Can you work these out from the model? Positions are in its coordinate system, mm. Face numbers are marked on the shaded views. A direction names the side the tool comes from. Round coordinates to 2 decimals unless told otherwise and drop trailing zeros. Write each loop counter-clockwise with the first axis right and the second up, starting at its lowest first coordinate (ties: lowest second). Pieces come first, ordered by that corner, then holes. Notation, with made-up numbers: M 79.25,8 L 97.25,8 A17 cw 97.25,41 Z; hole C 57,61.25 d10. An arc over 180 degrees is marked long. Answer in a Markdown table with one row per item. Add a question column.
(1) I'm going to push flat-ended pins straight in: pin 1 (2 mm diameter, centred on y = 4, z = -3, fed in from +X); pin 2 (1.5 mm diameter, centred on x = 15.5, z = -2, fed in from +Y); pin 3 (1.5 mm diameter, centred on x = 15, z = -3.5, fed in from -Y); pin 4 (1.5 mm diameter, centred on y = 5.5, z = -4, fed in from -X). Where does each tip first touch, or does it pass through?
(2) Suppose I cut it at A-A, the plane y = 0. Write out the boundary of the cut face in (x, z), then the cut area to 3 significant figures.
(3) For the marked faces 1, 2, 3, 4 and 5, which set-ups out of +Z, -Z, +X, -X, +Y, -Y let a thin tool reach every point of the face, with its end or its side?
(4) If we mould it in two halves opening along Y, with no side actions, what happens to the marked faces 6, 7 and 8? For each: released by +Y, released by -Y, zero draft, split by the parting line, or undercut.
(5) Suppose I cut it at D-D, the plane x = 8.5. Write out the boundary of the cut face in (y, z), then the cut area to 3 significant figures.
(6) Suppose I cut it at B-B, the plane x = 14.5. Write out the boundary of the cut face in (y, z), then the cut area to 3 significant figures.
(7) Suppose I cut it at C-C, the plane z = -2.56. Write out the boundary of the cut face in (x, y).
(8) If I drill on probe 1 along Y at (x, z) = (16.5, -3.6); probe 2 along X at (y, z) = (-3.6, -2.56); probe 3 along Z at (x, y) = (8, 2), over which ranges is the centre line in solid material (lowest first)?
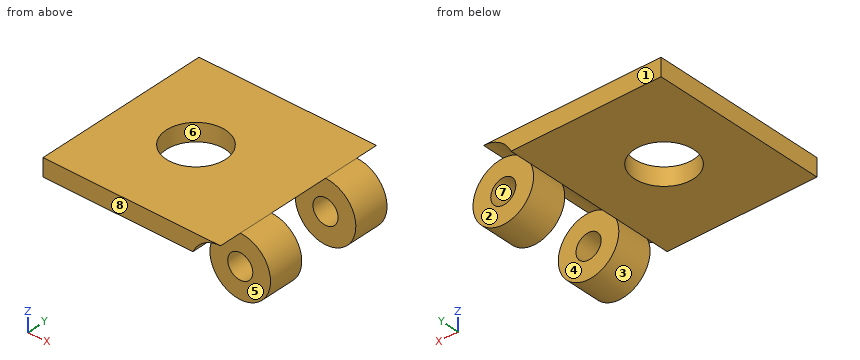
from build123d import *

# Parameters (mm, degrees)
BOSS_EXTRUDE1_DEPTH      = 7.5
BOSS_EXTRUDE1_DEPTH_BACK = 7.5
BOSS_EXTRUDE3_START      = 2.6
SKETCH1_4_R              = 2.56
SKETCH1_4_R_2            = 1.06
BOSS_EXTRUDE3_DEPTH      = 3
BOSS_EXTRUDE4_START      = -5.6
SKETCH1_5_R              = 2.56
SKETCH1_5_R_2            = 1.06
BOSS_EXTRUDE4_DEPTH      = 3
SKETCH2_R                = 2.5
CUT_EXTRUDE1_DEPTH       = 3


with BuildPart() as part:
    # Sketch1 → Boss-Extrude1 (new, two sides: drawn at the far end of the back side and taken through both)
    with BuildSketch(Plane(origin=(0, 0, 0), x_dir=(1, 0, 0), z_dir=(0, 1, 0)).offset(-BOSS_EXTRUDE1_DEPTH_BACK)):
        with BuildLine():
            Line((0, 1.5), (0, 0))
            Line((0, 0), (15, 0))
            ThreePointArc((15, 0), (13.614359354, 0.407420152), (12.66976396, 1.5))
            Line((12.66976396, 1.5), (0, 1.5))
        make_face()
    extrude(amount=BOSS_EXTRUDE1_DEPTH + BOSS_EXTRUDE1_DEPTH_BACK)

    # Sketch1_4 → Boss-Extrude3 (add)
    with BuildSketch(Plane(origin=(0, 0, 0), x_dir=(1, 0, 0), z_dir=(0, 1, 0)).offset(BOSS_EXTRUDE3_START)):
        with Locations((15, 2.56)):
            Circle(SKETCH1_4_R)
        with Locations(Location((15, 2.56, 0), (0, 0, 270))):
            Circle(SKETCH1_4_R_2, mode=Mode.SUBTRACT)
    extrude(amount=BOSS_EXTRUDE3_DEPTH)

    # Sketch1_5 → Boss-Extrude4 (add)
    with BuildSketch(Plane(origin=(0, 0, 0), x_dir=(1, 0, 0), z_dir=(0, 1, 0)).offset(BOSS_EXTRUDE4_START)):
        with Locations((15, 2.56)):
            Circle(SKETCH1_5_R)
        with Locations(Location((15, 2.56, 0), (0, 0, 270))):
            Circle(SKETCH1_5_R_2, mode=Mode.SUBTRACT)
    extrude(amount=BOSS_EXTRUDE4_DEPTH)

    # Sketch2 → Cut-Extrude1 (cut)
    with BuildSketch(Plane(origin=(0, 0, -1.5), x_dir=(-1, 0, 0), z_dir=(0, 0, -1))):
        with Locations((-6.33488198, 0)):
            Circle(SKETCH2_R)
    extrude(amount=-CUT_EXTRUDE1_DEPTH, mode=Mode.SUBTRACT)


solid = part.part
Calculated:
| question | item | result |
|---|---|---|
| 1 | pin 1 | x = 17.56 |
| 1 | pin 2 | y = 5.6 |
| 1 | pin 3 | y = -5.6 |
| 1 | pin 4 | x = 12.53 |
| 2 | outline | M 0,-1.5 L 3.83,-1.5 L 3.83,0 L 0,0 Z; M 8.83,-1.5 L 12.67,-1.5 A2.56 cw 15,0 L 8.83,0 Z |
| 2 | area | 12.5 mm² |
| 3 | face 1 | +Z, -Z, +X, -X, +Y |
| 3 | face 2 | -Z, +X, +Y |
| 3 | face 3 | +Y, -Y |
| 3 | face 4 | -Z, +X |
| 3 | face 5 | -Z, +X, -Y |
| 4 | face 6 | undercut |
| 4 | face 7 | zero draft |
| 4 | face 8 | released by -Y |
| 5 | outline | M -7.5,-1.5 L -1.25,-1.5 L -1.25,0 L -7.5,0 Z; M 1.25,-1.5 L 7.5,-1.5 L 7.5,0 L 1.25,0 Z |
| 5 | area | 18.8 mm² |
| 6 | outline | M -7.5,-0.05 L -5.6,-0.05 L -5.6,-1.63 L -2.6,-1.63 L -2.6,-0.05 L 2.6,-0.05 L 2.6,-1.63 L 5.6,-1.63 L 5.6,-0.05 L 7.5,-0.05 L 7.5,0 L -7.5,0 Z; M -5.6,-5.07 L -2.6,-5.07 L -2.6,-3.49 L -5.6,-3.49 Z; M 2.6,-5.07 L 5.6,-5.07 L 5.6,-3.49 L 2.6,-3.49 Z |
| 6 | area | 19.7 mm² |
| 7 | outline | M 12.44,-5.6 L 13.94,-5.6 L 13.94,-2.6 L 12.44,-2.6 Z; M 12.44,2.6 L 13.94,2.6 L 13.94,5.6 L 12.44,5.6 Z; M 16.06,-5.6 L 17.56,-5.6 L 17.56,-2.6 L 16.06,-2.6 Z; M 16.06,2.6 L 17.56,2.6 L 17.56,5.6 L 16.06,5.6 Z |
| 8 | probe 1 | -5.6 to -2.6, 2.6 to 5.6 |
| 8 | probe 2 | 12.44 to 13.94, 16.06 to 17.56 |
| 8 | probe 3 | -1.5 to 0 |
